Read the model definition and answer for the solid it produces. Units are mm, in the model's axes. Give positions to 0.01 mm unless a question says otherwise; leave off trailing zeros. Write each loop counter-clockwise with the first axis right and the second up, starting at its lowest first coordinate (ties: lowest second). Pieces come first, ordered by that corner, then holes. Notation, with made-up numbers: M -18,81 L -6,81 A17 ccw -6,101 Z; hole C -5,-15.5 d6. An arc over 180 degrees is marked long. Write each question's results on one line, items separated by ' | '. Start each with the question number.
```python
from build123d import *

# Parameters (mm, degrees)
SKETCH1_W           = 50.8
SKETCH1_H           = 25.4
SKETCH1_W_2         = 44.45
SKETCH1_H_2         = 19.05
BOSS_EXTRUDE1_DEPTH = 101.6
SKETCH3_R           = 2.4892
CUT_EXTRUDE2_DEPTH  = 26.4
SKETCH4_R           = 9.906
SKETCH4_R_2         = 2.4892
CUT_EXTRUDE3_DEPTH  = 51.8
SKETCH2_R           = 2.4892
CUT_EXTRUDE1_DEPTH  = 51.8
CUT_EXTRUDE4_REACH  = 27.4
SKETCH5_R           = 2.4892
CUT_EXTRUDE5_REACH  = 52.8
SKETCH7_R           = 2.4892


with BuildPart() as part:
    # Sketch1 → Boss-Extrude1 (new body, symmetric)
    with BuildSketch(Plane.XY):
        Rectangle(SKETCH1_W, SKETCH1_H)
        Rectangle(SKETCH1_W_2, SKETCH1_H_2, mode=Mode.SUBTRACT)
    extrude(amount=BOSS_EXTRUDE1_DEPTH, both=True)

    # Sketch3 → Cut-Extrude2 (cut, through all)
    with BuildSketch(Plane(origin=(0, 12.7, 0), x_dir=(1, 0, 0), z_dir=(0, 1, 0))):
        with Locations((-12.7, -93.6625)):
            Circle(SKETCH3_R)
        with Locations((0, -93.6625)):
            Circle(SKETCH3_R)
        with Locations((12.7, -93.6625)):
            Circle(SKETCH3_R)
        with Locations((12.7, 93.6625)):
            Circle(SKETCH3_R)
        with Locations((0, 93.6625)):
            Circle(SKETCH3_R)
        with Locations((-12.7, 93.6625)):
            Circle(SKETCH3_R)
    extrude(amount=-CUT_EXTRUDE2_DEPTH, mode=Mode.SUBTRACT)

    # Sketch4 → Cut-Extrude3 (cut, through all)
    with BuildSketch(Plane(origin=(25.4, 0, 0), x_dir=(0, 0, -1), z_dir=(1, 0, 0))):
        with Locations((-22.225, 0)):
            Circle(SKETCH4_R)
        with Locations((31.75, 0)):
            Circle(SKETCH4_R_2)
        with Locations((19.05, 0)):
            Circle(SKETCH4_R_2)
    extrude(amount=-CUT_EXTRUDE3_DEPTH, mode=Mode.SUBTRACT)

    # Sketch2 → Cut-Extrude1 (cut, through all)
    with BuildSketch(Plane(origin=(25.4, 0, 0), x_dir=(0, 0, -1), z_dir=(1, 0, 0))):
        with Locations((-93.6625, 0)):
            Circle(SKETCH2_R)
        with Locations((93.6625, 0)):
            Circle(SKETCH2_R)
        with Locations((-76.2, 0)):
            Circle(SKETCH2_R)
        with Locations((-63.5, 0)):
            Circle(SKETCH2_R)
        with Locations((63.5, 0)):
            Circle(SKETCH2_R)
        with Locations((76.2, 0)):
            Circle(SKETCH2_R)
    extrude(amount=-CUT_EXTRUDE1_DEPTH, mode=Mode.SUBTRACT)

    # Sketch5 → Cut-Extrude4 (cut, up to next)
    with BuildSketch(Plane.XZ.offset(12.7), mode=Mode.PRIVATE) as cut_extrude4_sk1:
        with Locations((-3.175, 66.675)):
            Circle(SKETCH5_R)
    cut_extrude4_tool1 = extrude(cut_extrude4_sk1.sketch, amount=-CUT_EXTRUDE4_REACH, mode=Mode.PRIVATE) & part.part
    add(cut_extrude4_tool1.solids().sort_by_distance((-3.175, -12.7, 66.675))[0], mode=Mode.SUBTRACT)
    # Sketch5 → Cut-Extrude4 (cut, up to next)
    with BuildSketch(Plane.XZ.offset(12.7), mode=Mode.PRIVATE) as cut_extrude4_sk2:
        with Locations((-15.875, 66.675)):
            Circle(SKETCH5_R)
    cut_extrude4_tool2 = extrude(cut_extrude4_sk2.sketch, amount=-CUT_EXTRUDE4_REACH, mode=Mode.PRIVATE) & part.part
    add(cut_extrude4_tool2.solids().sort_by_distance((-15.875, -12.7, 66.675))[0], mode=Mode.SUBTRACT)
    # Sketch5 → Cut-Extrude4 (cut, up to next)
    with BuildSketch(Plane.XZ.offset(12.7), mode=Mode.PRIVATE) as cut_extrude4_sk3:
        with Locations((-15.875, 53.975)):
            Circle(SKETCH5_R)
    cut_extrude4_tool3 = extrude(cut_extrude4_sk3.sketch, amount=-CUT_EXTRUDE4_REACH, mode=Mode.PRIVATE) & part.part
    add(cut_extrude4_tool3.solids().sort_by_distance((-15.875, -12.7, 53.975))[0], mode=Mode.SUBTRACT)
    # Sketch5 → Cut-Extrude4 (cut, up to next)
    with BuildSketch(Plane.XZ.offset(12.7), mode=Mode.PRIVATE) as cut_extrude4_sk4:
        with Locations((-3.175, 53.975)):
            Circle(SKETCH5_R)
    cut_extrude4_tool4 = extrude(cut_extrude4_sk4.sketch, amount=-CUT_EXTRUDE4_REACH, mode=Mode.PRIVATE) & part.part
    add(cut_extrude4_tool4.solids().sort_by_distance((-3.175, -12.7, 53.975))[0], mode=Mode.SUBTRACT)
    # Sketch5 → Cut-Extrude4 (cut, up to next)
    with BuildSketch(Plane.XZ.offset(12.7), mode=Mode.PRIVATE) as cut_extrude4_sk5:
        with Locations((-3.175, -9.525)):
            Circle(SKETCH5_R)
    cut_extrude4_tool5 = extrude(cut_extrude4_sk5.sketch, amount=-CUT_EXTRUDE4_REACH, mode=Mode.PRIVATE) & part.part
    add(cut_extrude4_tool5.solids().sort_by_distance((-3.175, -12.7, -9.525))[0], mode=Mode.SUBTRACT)
    # Sketch5 → Cut-Extrude4 (cut, up to next)
    with BuildSketch(Plane.XZ.offset(12.7), mode=Mode.PRIVATE) as cut_extrude4_sk6:
        with Locations((-15.875, -9.525)):
            Circle(SKETCH5_R)
    cut_extrude4_tool6 = extrude(cut_extrude4_sk6.sketch, amount=-CUT_EXTRUDE4_REACH, mode=Mode.PRIVATE) & part.part
    add(cut_extrude4_tool6.solids().sort_by_distance((-15.875, -12.7, -9.525))[0], mode=Mode.SUBTRACT)
    # Sketch5 → Cut-Extrude4 (cut, up to next)
    with BuildSketch(Plane.XZ.offset(12.7), mode=Mode.PRIVATE) as cut_extrude4_sk7:
        with Locations((-15.875, -22.225)):
            Circle(SKETCH5_R)
    cut_extrude4_tool7 = extrude(cut_extrude4_sk7.sketch, amount=-CUT_EXTRUDE4_REACH, mode=Mode.PRIVATE) & part.part
    add(cut_extrude4_tool7.solids().sort_by_distance((-15.875, -12.7, -22.225))[0], mode=Mode.SUBTRACT)
    # Sketch5 → Cut-Extrude4 (cut, up to next)
    with BuildSketch(Plane.XZ.offset(12.7), mode=Mode.PRIVATE) as cut_extrude4_sk8:
        with Locations((-3.175, -22.225)):
            Circle(SKETCH5_R)
    cut_extrude4_tool8 = extrude(cut_extrude4_sk8.sketch, amount=-CUT_EXTRUDE4_REACH, mode=Mode.PRIVATE) & part.part
    add(cut_extrude4_tool8.solids().sort_by_distance((-3.175, -12.7, -22.225))[0], mode=Mode.SUBTRACT)

    # Sketch7 → Cut-Extrude5 (cut, up to next)
    with BuildSketch(Plane(origin=(25.4, 0, 0), x_dir=(0, 0, -1), z_dir=(1, 0, 0)), mode=Mode.PRIVATE) as cut_extrude5_sk1:
        with Locations((44.45, 0)):
            Circle(SKETCH7_R)
    cut_extrude5_tool1 = extrude(cut_extrude5_sk1.sketch, amount=-CUT_EXTRUDE5_REACH, mode=Mode.PRIVATE) & part.part
    add(cut_extrude5_tool1.solids().sort_by_distance((25.4, 0, -44.45))[0], mode=Mode.SUBTRACT)
    # Sketch7 → Cut-Extrude5 (cut, up to next)
    with BuildSketch(Plane(origin=(25.4, 0, 0), x_dir=(0, 0, -1), z_dir=(1, 0, 0)), mode=Mode.PRIVATE) as cut_extrude5_sk2:
        with Locations((6.35, 0)):
            Circle(SKETCH7_R)
    cut_extrude5_tool2 = extrude(cut_extrude5_sk2.sketch, amount=-CUT_EXTRUDE5_REACH, mode=Mode.PRIVATE) & part.part
    add(cut_extrude5_tool2.solids().sort_by_distance((25.4, 0, -6.35))[0], mode=Mode.SUBTRACT)
    # Sketch7 → Cut-Extrude5 (cut, up to next)
    with BuildSketch(Plane(origin=(25.4, 0, 0), x_dir=(0, 0, -1), z_dir=(1, 0, 0)), mode=Mode.PRIVATE) as cut_extrude5_sk3:
        with Locations((-6.35, 0)):
            Circle(SKETCH7_R)
    cut_extrude5_tool3 = extrude(cut_extrude5_sk3.sketch, amount=-CUT_EXTRUDE5_REACH, mode=Mode.PRIVATE) & part.part
    add(cut_extrude5_tool3.solids().sort_by_distance((25.4, 0, 6.35))[0], mode=Mode.SUBTRACT)
    # Sketch7 → Cut-Extrude5 (cut, up to next)
    with BuildSketch(Plane(origin=(25.4, 0, 0), x_dir=(0, 0, -1), z_dir=(1, 0, 0)), mode=Mode.PRIVATE) as cut_extrude5_sk4:
        with Locations((-41.275, 0)):
            Circle(SKETCH7_R)
    cut_extrude5_tool4 = extrude(cut_extrude5_sk4.sketch, amount=-CUT_EXTRUDE5_REACH, mode=Mode.PRIVATE) & part.part
    add(cut_extrude5_tool4.solids().sort_by_distance((25.4, 0, 41.275))[0], mode=Mode.SUBTRACT)


solid = part.part
```
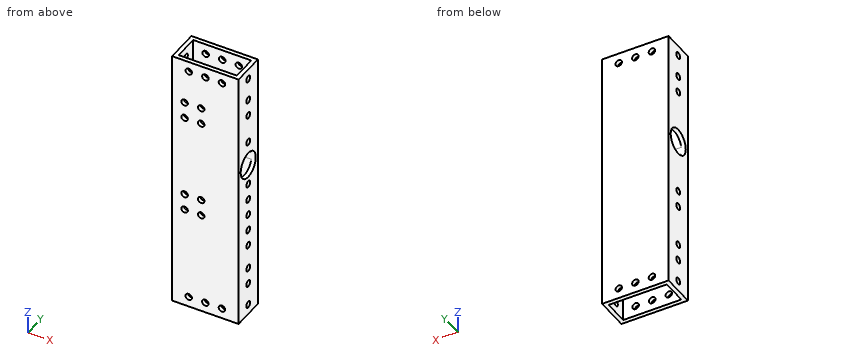
Item 1: Section C-C, the plane y = -6.5 is taken. Determine the outline of the cut face in (x, z) (3 decimals), then the cut area to 3 significant figures.
Item 2: Section A-A, the plane x = 12.7 is taken. Determine the outline of the cut face in (y, z) (3 decimals).
Item 3: Section D-D, the plane x = 4.5 is taken. Determine the outline of the cut face in (y, z) (3 decimals).
Item 4: Given P1, Ø5.5, axis at y = 0, z = 76.2, coming from the -X side; P2, Ø4, axis at x = 12.7, z = -93.66, coming from the -Y side, each flat-ended and moving along its own axis, determine where each tip first touches the part or whether it passes through.
Item 5: Section B-B, the plane z = -63.5 is taken. Determine the outline of the cut face in (x, y) (3 decimals), then the cut area to 3 significant figures.
Item 6: Straight lines are drawn through the part: line 1 (Z direction, x = -12.7, y = -10.8); line 2 (Y direction, x = -21, z = 49) (3 decimals); line 3 (X direction, y = -6.75, z = 68) (3 decimals). For each, find the intervals that lie inside material, in ascending order.
Worked out:
1) outline: M -25.4,-101.6 L -22.225,-101.6 L -22.225,14.75 L -25.4,14.75 Z; M -25.4,29.7 L -22.225,29.7 L -22.225,101.6 L -25.4,101.6 Z; M 22.225,-101.6 L 25.4,-101.6 L 25.4,14.75 L 22.225,14.75 Z; M 22.225,29.7 L 25.4,29.7 L 25.4,101.6 L 22.225,101.6 Z | area: 1,200 mm²
2) outline: M -12.7,-101.6 L -9.525,-101.6 L -9.525,-96.152 L -12.7,-96.152 Z; M -12.7,-91.173 L -9.525,-91.173 L -9.525,19.504 A9.906 cw -9.525,24.946 L -9.525,91.173 L -12.7,91.173 Z; M -12.7,96.152 L -9.525,96.152 L -9.525,101.6 L -12.7,101.6 Z; M 9.525,-101.6 L 12.7,-101.6 L 12.7,-96.152 L 9.525,-96.152 Z; M 9.525,-91.173 L 12.7,-91.173 L 12.7,91.173 L 9.525,91.173 L 9.525,24.946 A9.906 cw 9.525,19.504 Z; M 9.525,96.152 L 12.7,96.152 L 12.7,101.6 L 9.525,101.6 Z
3) outline: M -12.7,-101.6 L -9.525,-101.6 L -9.525,19.504 A9.906 cw -9.525,24.946 L -9.525,101.6 L -12.7,101.6 Z; M 9.525,-101.6 L 12.7,-101.6 L 12.7,101.6 L 9.525,101.6 L 9.525,24.946 A9.906 cw 9.525,19.504 Z
4) P1: stops at x = -25.4 | P2: passes through
5) outline: M -25.4,-12.7 L 25.4,-12.7 L 25.4,-2.489 L 22.225,-2.489 L 22.225,-9.525 L -22.225,-9.525 L -22.225,-2.489 L -25.4,-2.489 Z; M -25.4,2.489 L -22.225,2.489 L -22.225,9.525 L 22.225,9.525 L 22.225,2.489 L 25.4,2.489 L 25.4,12.7 L -25.4,12.7 Z | area: 412 mm²
6) line 1: z = -101.6 to -96.15, -91.17 to 91.17, 96.15 to 101.6 | line 2: y = -12.7 to -9.525, 9.525 to 12.7 | line 3: x = -25.4 to -22.225, 22.225 to 25.4
